```python
from build123d import *

# Parameters (mm, degrees)
F0_R     = 3
F1_DEPTH = 1
F2_R     = 0.5
F3_R     = 2
F4_DEPTH = 75


with BuildPart() as f1:
    # F0 (on Top) → F1 (new body)
    with BuildSketch(Plane.XY):
        Circle(F0_R)
    extrude(amount=F1_DEPTH)

    # F2
    f2_edges = [f1.edges().sort_by_distance(p)[0] for p in [
        (-3, 0, 1),
    ]]
    fillet(f2_edges, radius=F2_R)

    # F3 (on face) → F4 (join)
    with BuildSketch(Plane(origin=(0, 0, 0), x_dir=(1, 0, 0), z_dir=(0, 0, -1))):
        Circle(F3_R)
    extrude(amount=F4_DEPTH)


solid = f1.part
```
Can you work these out from the model? Positions are in its coordinate system, mm. A direction names the side the tool comes from. Coordinates: 2 decimals unless noted, no trailing zeros. Loops run counter-clockwise (first coordinate to the right, second up) from the corner with the lowest first, then second, coordinate; pieces in that order, holes last.
1) For pin 1 (1 mm diameter, centred on x = -1.5, z = -23, fed in from -Y), with a flat end and sliding along its axis, tell me the tip position at first contact or that it passes through.
2) I need wall thicknesses on probe 1 along Z at (x, y) = (0.4, -2.15); probe 2 along X at (y, z) = (0.2, -52); probe 3 along Y at (x, z) = (-1.1, -52). Which ranges of each line are inside material? Lowest first, please.
3) Which directions (+Z, -Z, +X, -X, +Y, -Y) give clear straight access to the entire face, cutting with the end or side of a thin tool? Please do faces 1 (the flat face through (0, 0, 1)), 2 (the cylindrical face through (0, 2, -37)).
4) Imagine slicing it at A-A on x = 0. List the corners of the cut face in (y, z) for me, plus the area to 3 significant figures.
5) Imagine slicing it at C-C on z = -35. List the corners of the cut face in (x, y) for me.
Completed:
1. pin 1: stops at y = -1.73
2. probe 1: z = 0 to 1
2. probe 2: x = -1.99 to 1.99
2. probe 3: y = -1.67 to 1.67
3. face 1: +Z, +X, -X, +Y, -Y
3. face 2: -Z
4. outline: (-3, 0) - (-2, 0) - (-2, -75) - (2, -75) - (2, 0) - (3, 0) - (3, 0.5) arc R0.5 ccw to (2.5, 1) - (-2.5, 1) arc R0.5 ccw to (-3, 0.5) - close
4. area: 306 mm2
5. outline: circle Ø4 at (0, 0)
